Work out the finished part from the listing and answer in its coordinate system (mm). Face numbers are marked on the shaded views. Coordinates: 2 decimals unless noted, no trailing zeros. Write each loop counter-clockwise with the first axis right and the second up, starting at its lowest first coordinate (ties: lowest second). Pieces come first, ordered by that corner, then holes. Notation, with made-up numbers: (-16.5, -25.75) - (20.5, -25.75) arc R22 ccw to (20.5, 13.25) - close; hole circle Ø11 at (10.25, 15). An arc over 180 degrees is marked (long way). Use a Markdown table: item, result. Add a question column.
(1) The part is cut by section A-A, the plane z = -4.75. Give the vertices of the cut face in (x, y), then the cut area to 3 significant figures.
(2) Given pin 1 Ø4 at (y, z) = (4.5, -12.5) entering from -X; pin 2 Ø2 at (y, z) = (0, -12) entering from +X; pin 3 Ø6 at (y, z) = (-4, -6) entering from -X, each flat-ended and moving along its own axis, determine where each tip first touches the part or whether it passes through.
(3) Find the intervals of material crossed by line 1 (Y direction, x = 0, z = -7.75); line 2 (Y direction, x = 0, z = -0.75); line 3 (Z direction, x = -0.5, y = -1.75), in increasing order. Write a range as from..to.
(4) For a pull along X with two mould halves and no side action, classify the marked faces 1, 2 and 3 as released by +X, released by -X, zero draft, split by the parting line, or undercut.
from build123d import *

# Parameters (mm, degrees)
CROQUIS1_W            = 5.9
CROQUIS1_H            = 14.8
CROQUIS2_R            = 2.1
CORTAR_EXTRUIR2_DEPTH = 13
CROQUIS23_W           = 1.5
CROQUIS23_H           = 13.3
REDONDEO1_R           = 0.2
REDONDEO2_R           = 1.7
REDONDEO3_R           = 1.7


with BuildPart() as part:
    # Croquis1 → Revolución1 (revolve)
    with BuildSketch(Plane(origin=(0, 0, 0), x_dir=(1, 0, 0), z_dir=(0, 1, 0))):
        with Locations((2.95, 7.4)):
            Rectangle(CROQUIS1_W, CROQUIS1_H)
    revolve(axis=Axis((0, 0, 0), (0, 0, -1)))

    # Croquis2 → Cortar-Extruir2 (cut)
    with BuildSketch(Plane.XY):
        Circle(CROQUIS2_R)
    extrude(amount=-CORTAR_EXTRUIR2_DEPTH, mode=Mode.SUBTRACT)

    # Croquis23 → Cortar-Revolución2 (revolve, cut)
    with BuildSketch(Plane(origin=(0, 0, 0), x_dir=(1, 0, 0), z_dir=(0, 1, 0))):
        with Locations((5.15, 8.15)):
            Rectangle(CROQUIS23_W, CROQUIS23_H)
    revolve(axis=Axis((0, 0, -1.5), (0, 0, -1)), mode=Mode.SUBTRACT)

    # Redondeo1
    redondeo1_edges = [part.edges().sort_by_distance(p)[0] for p in [
        (-5.9, 0, -1.5),
    ]]
    fillet(redondeo1_edges, radius=REDONDEO1_R)

    # Redondeo2
    redondeo2_edges = [part.edges().sort_by_distance(p)[0] for p in [
        (-4.4, 0, -14.8),
    ]]
    fillet(redondeo2_edges, radius=REDONDEO2_R)

    # Redondeo3
    redondeo3_edges = [part.edges().sort_by_distance(p)[0] for p in [
        (-4.4, 0, -1.5),
    ]]
    fillet(redondeo3_edges, radius=REDONDEO3_R)


solid = part.part
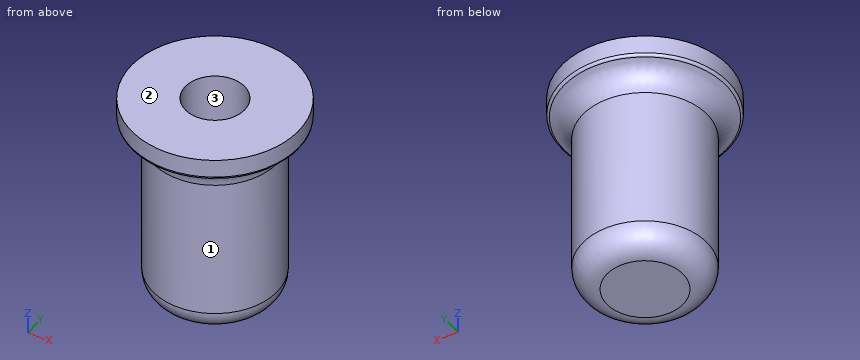
Model answer:
| question | item | result |
|---|---|---|
| 1 | outline | circle Ø8.8 at (0, 0); hole circle Ø4.2 at (0, 0) |
| 1 | area | 47.0 mm^2 |
| 2 | pin 1 | x = -3.62 |
| 2 | pin 2 | x = 4.4 |
| 2 | pin 3 | x = -4.28 |
| 3 | line 1 | -4.4..-2.1, 2.1..4.4 |
| 3 | line 2 | -5.9..-2.1, 2.1..5.9 |
| 3 | line 3 | -14.8..-13 |
| 4 | face 1 | split by the parting line |
| 4 | face 2 | zero draft |
| 4 | face 3 | undercut |
